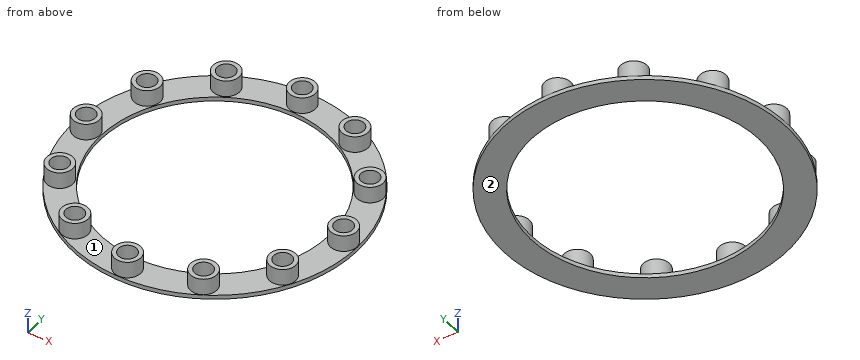
from build123d import *

# Parameters (mm, degrees)
F0_R     = 102.5
F0_R_2   = 9.5
F0_R_3   = 82.5
F1_DEPTH = 3
F0_R_4   = 6.5
F2_DEPTH = 15
F3_DEPTH = 2


with BuildPart() as f1:
    # F0 (on Top) → F1 (new body)
    with BuildSketch(Plane.XY):
        Circle(F0_R)
        with Locations((-46.328817, -80.243864)):
            Circle(F0_R_2, mode=Mode.SUBTRACT)
        with Locations((-80.243864, -46.328817)):
            Circle(F0_R_2, mode=Mode.SUBTRACT)
        with Locations((0, -92.657633)):
            Circle(F0_R_2, mode=Mode.SUBTRACT)
        with Locations((46.328817, -80.243864)):
            Circle(F0_R_2, mode=Mode.SUBTRACT)
        with Locations((80.243864, -46.328817)):
            Circle(F0_R_2, mode=Mode.SUBTRACT)
        with Locations((-92.657633, 0)):
            Circle(F0_R_2, mode=Mode.SUBTRACT)
        with Locations((-80.243864, 46.328817)):
            Circle(F0_R_2, mode=Mode.SUBTRACT)
        with Locations((-46.328817, 80.243864)):
            Circle(F0_R_2, mode=Mode.SUBTRACT)
        Circle(F0_R_3, mode=Mode.SUBTRACT)
        with Locations((92.657633, 0)):
            Circle(F0_R_2, mode=Mode.SUBTRACT)
        with Locations((80.243864, 46.328817)):
            Circle(F0_R_2, mode=Mode.SUBTRACT)
        with Locations((0, 92.657633)):
            Circle(F0_R_2, mode=Mode.SUBTRACT)
        with Locations((46.328817, 80.243864)):
            Circle(F0_R_2, mode=Mode.SUBTRACT)
    extrude(amount=F1_DEPTH)

    # F0 (on Top) → F2 (join)
    with BuildSketch(Plane.XY):
        with Locations((-80.243864, 46.328817)):
            Circle(F0_R_2)
        with Locations((-80.243864, 46.328817)):
            Circle(F0_R_4, mode=Mode.SUBTRACT)
        with Locations((-46.328817, 80.243864)):
            Circle(F0_R_2)
        with Locations((-46.328817, 80.243864)):
            Circle(F0_R_4, mode=Mode.SUBTRACT)
        with Locations((0, 92.657633)):
            Circle(F0_R_2)
        with Locations((0, 92.657633)):
            Circle(F0_R_4, mode=Mode.SUBTRACT)
        with Locations((92.657633, 0)):
            Circle(F0_R_2)
        with Locations((92.657633, 0)):
            Circle(F0_R_4, mode=Mode.SUBTRACT)
        with Locations((80.243864, -46.328817)):
            Circle(F0_R_2)
        with Locations((80.243864, -46.328817)):
            Circle(F0_R_4, mode=Mode.SUBTRACT)
        with Locations((46.328817, -80.243864)):
            Circle(F0_R_2)
        with Locations((46.328817, -80.243864)):
            Circle(F0_R_4, mode=Mode.SUBTRACT)
        with Locations((0, -92.657633)):
            Circle(F0_R_2)
        with Locations((0, -92.657633)):
            Circle(F0_R_4, mode=Mode.SUBTRACT)
        with Locations((-46.328817, -80.243864)):
            Circle(F0_R_2)
        with Locations((-46.328817, -80.243864)):
            Circle(F0_R_4, mode=Mode.SUBTRACT)
        with Locations((-80.243864, -46.328817)):
            Circle(F0_R_2)
        with Locations((-80.243864, -46.328817)):
            Circle(F0_R_4, mode=Mode.SUBTRACT)
        with Locations((-92.657633, 0)):
            Circle(F0_R_2)
        with Locations((-92.657633, 0)):
            Circle(F0_R_4, mode=Mode.SUBTRACT)
        with Locations((46.328817, 80.243864)):
            Circle(F0_R_2)
        with Locations((46.328817, 80.243864)):
            Circle(F0_R_4, mode=Mode.SUBTRACT)
        with Locations((80.243864, 46.328817)):
            Circle(F0_R_2)
        with Locations((80.243864, 46.328817)):
            Circle(F0_R_4, mode=Mode.SUBTRACT)
    extrude(amount=F2_DEPTH)

    # F0 (on Top) → F3 (join)
    with BuildSketch(Plane.XY):
        with Locations((-46.328817, 80.243864)):
            Circle(F0_R_4)
        with Locations((0, 92.657633)):
            Circle(F0_R_4)
        with Locations((92.657633, 0)):
            Circle(F0_R_4)
        with Locations((80.243864, -46.328817)):
            Circle(F0_R_4)
        with Locations((46.328817, -80.243864)):
            Circle(F0_R_4)
        with Locations((0, -92.657633)):
            Circle(F0_R_4)
        with Locations((-46.328817, -80.243864)):
            Circle(F0_R_4)
        with Locations((-80.243864, -46.328817)):
            Circle(F0_R_4)
        with Locations((-92.657633, 0)):
            Circle(F0_R_4)
        with Locations((-80.243864, 46.328817)):
            Circle(F0_R_4)
        with Locations((46.328817, 80.243864)):
            Circle(F0_R_2)
        with Locations((46.328817, 80.243864)):
            Circle(F0_R_4, mode=Mode.SUBTRACT)
        with Locations((80.243864, 46.328817)):
            Circle(F0_R_2)
        with Locations((80.243864, 46.328817)):
            Circle(F0_R_4, mode=Mode.SUBTRACT)
        with Locations((46.328817, 80.243864)):
            Circle(F0_R_4)
        with Locations((80.243864, 46.328817)):
            Circle(F0_R_4)
    extrude(amount=F3_DEPTH)


solid = f1.part
Design review of the part built by this model. Coordinates are the model's own, in mm. Face numbers are marked on the shaded views. Give positions to 0.01 mm unless a question says otherwise; leave off trailing zeros. Loops run counter-clockwise (first coordinate to the right, second up) from the corner with the lowest first, then second, coordinate; pieces in that order, holes last. Notation, with made-up numbers: (14.5, -28) - (69.5, -28) arc R22 ccw to (69.5, -22) - close; hole circle Ø9 at (-13.5, 57). An arc over 180 degrees is marked (long way). Write item = value, one per line.
1) Take a section at D-D on x = 76.5. State the section outline as (y, z) points.
Result sheet:
outline = (-68.22, 0) - (-30.89, 0) - (-30.89, 3) - (-37.6, 3) - (-37.6, 15) - (-41.02, 15) - (-41.02, 2) - (-51.64, 2) - (-51.64, 15) - (-55.06, 15) - (-55.06, 3) - (-68.22, 3) - close; (30.89, 0) - (68.22, 0) - (68.22, 3) - (55.06, 3) - (55.06, 15) - (51.64, 15) - (51.64, 2) - (41.02, 2) - (41.02, 15) - (37.6, 15) - (37.6, 3) - (30.89, 3) - close
2) Take a section at A-A on x = 0. State the section outline as (y, z) points, and give its area (3 significant figures).
Result sheet:
outline = (-102.5, 0) - (-82.5, 0) - (-82.5, 3) - (-83.16, 3) - (-83.16, 15) - (-86.16, 15) - (-86.16, 2) - (-99.16, 2) - (-99.16, 15) - (-102.16, 15) - (-102.16, 3) - (-102.5, 3) - close; (82.5, 0) - (102.5, 0) - (102.5, 3) - (102.16, 3) - (102.16, 15) - (99.16, 15) - (99.16, 2) - (86.16, 2) - (86.16, 15) - (83.16, 15) - (83.16, 3) - (82.5, 3) - close
area = 238 mm2
3) Take a section at C-C on z = 9.25. Count the separate pieces of the cut face and the enclosed holes in it, and give its area (3 significant figures).
Result sheet:
separate_pieces = 12
enclosed_holes = 12
area = 1,810 mm2
4) Take a section at B-B on y = -32. State the section outline as (x, z) points, and give its area (3 significant figures).
Result sheet:
outline = (-97.38, 0) - (-76.04, 0) - (-76.04, 3) - (-97.38, 3) - close; (76.04, 0) - (97.38, 0) - (97.38, 3) - (76.04, 3) - close
area = 128 mm2
5) Clearance check with flat-ended pins moving along their axes: pin 1 Ø1 at (y, z) = (-43, 12.5) entering from -X; pin 2 Ø6 at (y, z) = (-14, 5) entering from -X; pin 3 Ø5 at (x, z) = (11.5, 4.5) entering from -Y. State where each tip first meets the part, or that it passes through.
Result sheet:
pin_1 = -89.31
pin_2 = -101.82
pin_3 = -102.06
6) Draft analysis for pull direction X (two halves, no side actions). For the marked faces 1 and 2, state which applies: +X half, -X half, draft (parallel to the pull), parting line (faces both ways), or undercut.
Result sheet:
face_1 = undercut
face_2 = draft
7) To check wall thickness, follow line 1 (Y direction, x = 46.5, z = 9); line 2 (Y direction, x = 0, z = 9.25); line 3 (X direction, y = 3, z = 6.25). State the ranges of each line that lie inside material, in increasing order.
Result sheet:
line_1 = -89.74 to -86.74, -73.75 to -70.75, 70.75 to 73.75, 86.74 to 89.74
line_2 = -102.16 to -99.16, -86.16 to -83.16, 83.16 to 86.16, 99.16 to 102.16
line_3 = -101.67 to -98.42, -86.89 to -83.64, 83.64 to 86.89, 98.42 to 101.67
